```python
from build123d import *

# Parameters (mm, degrees)
SKETCH1_W           = 67.125
SKETCH1_H           = 30
BOSS_EXTRUDE1_DEPTH = 30
SKETCH2_W           = 57.125
SKETCH2_H           = 25
CUT_EXTRUDE1_DEPTH  = 25
SKETCH3_R           = 2.75
CUT_EXTRUDE2_DEPTH  = 76.038427655


with BuildPart() as part:
    # Sketch1 → Boss-Extrude1 (new body)
    with BuildSketch(Plane.XY):
        Rectangle(SKETCH1_W, SKETCH1_H)
    extrude(amount=BOSS_EXTRUDE1_DEPTH)

    # Sketch2 → Cut-Extrude1 (cut)
    with BuildSketch(Plane(origin=(0, 0, 0), x_dir=(-1, 0, 0), z_dir=(0, 0, -1))):
        with Locations((0, 2.5)):
            Rectangle(SKETCH2_W, SKETCH2_H)
    extrude(amount=-CUT_EXTRUDE1_DEPTH, mode=Mode.SUBTRACT)

    # Sketch3 → Cut-Extrude2 (cut, through all)
    with BuildSketch(Plane(origin=(33.5625, 0, 0), x_dir=(0, 0, -1), z_dir=(1, 0, 0))):
        with Locations((-15, 0)):
            Circle(SKETCH3_R)
    extrude(amount=-CUT_EXTRUDE2_DEPTH, mode=Mode.SUBTRACT)


solid = part.part
```
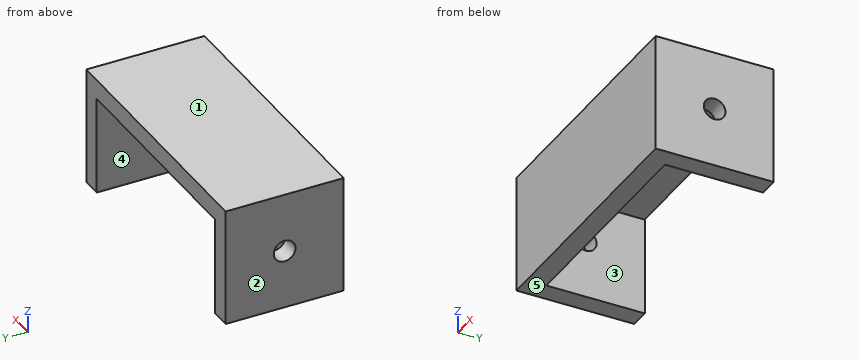
The listing builds one solid part. Answer for the finished solid, in the listing's coordinates (mm). Face numbers are marked on the shaded views. A direction names the side the tool comes from. Coordinates: 2 decimals unless noted, no trailing zeros. Loops run counter-clockwise (first coordinate to the right, second up) from the corner with the lowest first, then second, coordinate; pieces in that order, holes last. Notation, with made-up numbers: M 40.25,-8 L 95.25,-8 A36 ccw 95.25,26 Z; hole C -23.5,-10 d1. An arc over 180 degrees is marked long. Answer as a JSON object with one key per item and string values. Group by question number.
Item 1: Section B-B (z = 15) is taken. Write down the section's boundary in (x, y).
Item 2: Each of these flat-tipped pins is pushed along its axis until it touches: P1, Ø1.5, axis at x = -2.5, y = 6.5, coming from the -Z side; P2, Ø1.5, axis at x = 20, z = 17.5, coming from the +Y side; P3, Ø3.5, axis at y = 0, z = 15, coming from the +X side. Where does it stop, or does it pass through?
Item 3: Determine the mould class of the marked faces 1, 2 and 3 for opening direction X: +X half, -X half, draft (parallel to the pull), parting line (faces both ways), or undercut.
Item 4: Section A-A (y = 0) is taken. Write down the section's boundary in (x, z), and give its area (3 significant figures).
Item 5: Which of the six approach directions +Z, -Z, +X, -X, +Y, -Y give full straight-line access (tool end or side, diameter ignored) to the marked faces 4 and 5?
Item 6: Section C-C (z = 5.5) is taken. Write down the section's boundary in (x, y), and give its area (3 significant figures).
Item 7: Consider L1, parallel to X at y = 2.75, z = 3.75; L2, parallel to Y at x = -31.25, z = 15; L3, parallel to Z at x = -1.5, y = 13. Determine where each line is inside the solid, lowest interval first.
Item 8: Section D-D (y = -4) is taken. Write down the section's boundary in (x, z).
Solved:
{
 "1": {"outline": "M -33.56,-15 L 33.56,-15 L 33.56,-2.75 L 28.56,-2.75 L 28.56,-10 L -28.56,-10 L -28.56,-2.75 L -33.56,-2.75 Z; M -33.56,2.75 L -28.56,2.75 L -28.56,15 L -33.56,15 Z; M 28.56,2.75 L 33.56,2.75 L 33.56,15 L 28.56,15 Z"},
 "2": {"P1": "stops at z = 25", "P2": "stops at y = -10", "P3": "passes through"},
 "3": {"face 1": "draft", "face 2": "-X half", "face 3": "undercut"},
 "4": {"outline": "M -33.56,0 L -28.56,0 L -28.56,12.25 L -33.56,12.25 Z; M -33.56,17.75 L -28.56,17.75 L -28.56,25 L 28.56,25 L 28.56,17.75 L 33.56,17.75 L 33.56,30 L -33.56,30 Z; M 28.56,0 L 33.56,0 L 33.56,12.25 L 28.56,12.25 Z", "area": "531 mm2"},
 "5": {"face 4": "-Z, +Y", "face 5": "-Z, +X, -X, +Y, -Y"},
 "6": {"outline": "M -33.56,-15 L 33.56,-15 L 33.56,15 L 28.56,15 L 28.56,-10 L -28.56,-10 L -28.56,15 L -33.56,15 Z", "area": "586 mm2"},
 "7": {"L1": "x = -33.56 to -28.56, 28.56 to 33.56", "L2": "y = -15 to -2.75, 2.75 to 15", "L3": "z = 25 to 30"},
 "8": {"outline": "M -33.56,0 L -28.56,0 L -28.56,25 L 28.56,25 L 28.56,0 L 33.56,0 L 33.56,30 L -33.56,30 Z"}
}
